The model under review builds one solid part; all positions refer to its coordinate system, in mm. Face numbers are marked on the shaded views. A direction names the side the tool comes from. Round coordinates to 2 decimals unless told otherwise and drop trailing zeros. Order: outer loops, then holes, each group sorted by start corner. A loop starts at its lowest first (then second) coordinate and runs counter-clockwise, first axis right, second up. Notation, with made-up numbers: M 50.5,70.5 L 59.5,70.5 A15 ccw 59.5,92.5 Z; hole C 56,34.5 d1. An arc over 180 degrees is marked long. Answer as a JSON object with one key per item and string values. Group by question number.
1) Consider section C-C, the plane x = 8. Write out the cut boundary in (y, z) (3 decimals), then the cut area to 3 significant figures.
2) For the marked faces 4, 5 and 6, list the 3-axis set-ups (+Z, -Z, +X, -X, +Y, -Y) from which the entire face can be reached by the end or side of a thin tool; tool diameter is ignored.
3) Consider section B-B, the plane z = 0. Write out the cut boundary in (x, y), then the cut area to 3 significant figures.
4) To check wall thickness, follow line 1 (X direction, y = 3.75, z = 0); line 2 (Z direction, x = 29, y = 6); line 3 (X direction, y = 2.5, z = 3). State the ranges of each line that lie inside material, in increasing order.
5) Consider section A-A, the plane y = 4. Write out the cut boundary in (x, z) (1 decimal), then the cut area to 3 significant figures.
6) The part is to be moulded in two halves that separate along X. For the marked faces 1, 2 and 3, say which applies: +X half, -X half, draft (parallel to the pull), parting line (faces both ways), or undercut.
7) Insertion check: pin 1 Ø3.5 at (x, y) = (16, 5) entering from +Z (3 decimals); pin 2 Ø2 at (x, z) = (18.5, 4) entering from -Y; pin 3 Ø5.5 at (x, z) = (29, 0) entering from +Y; pin 4 Ø1 at (x, y) = (14.5, 5.5) entering from -Z (3 decimals). Each pin has a flat end and moves straight along its axis. Give the tip position at first contact, or say it passes through.
```python
from build123d import *

# Parameters (mm, degrees)
SKETCH1_R           = 5
BOSS_EXTRUDE1_DEPTH = 10
FILLET1_R           = 2.54
SCALE1_SCALE        = 0.66


with BuildPart() as part:
    # Sketch1 → Boss-Extrude1 (new body)
    with BuildSketch(Plane(origin=(0, 0, 0), x_dir=(1, 0, 0), z_dir=(0, 1, 0))):
        with BuildLine():
            Line((-0.840776184, -6.25), (25.840776184, -6.25))
            ThreePointArc((25.840776184, -6.25), (28.902638362, -6.730283618), (31.670388092, -8.125))
            ThreePointArc((31.670388092, -8.125), (47.5, 0), (31.670388092, 8.125))
            ThreePointArc((31.670388092, 8.125), (28.902638362, 6.730283618), (25.840776184, 6.25))
            Line((25.840776184, 6.25), (-0.840776184, 6.25))
            ThreePointArc((-0.840776184, 6.25), (-3.902638362, 6.730283618), (-6.670388092, 8.125))
            ThreePointArc((-6.670388092, 8.125), (-22.5, 0), (-6.670388092, -8.125))
            ThreePointArc((-6.670388092, -8.125), (-3.902638362, -6.730283618), (-0.840776184, -6.25))
        make_face()
        with Locations((-12.5, 0)):
            Circle(SKETCH1_R, mode=Mode.SUBTRACT)
        with Locations((37.5, 0)):
            Circle(SKETCH1_R, mode=Mode.SUBTRACT)
    extrude(amount=BOSS_EXTRUDE1_DEPTH)

    # Fillet1
    fillet1_edges = [part.edges().sort_by_distance(p)[0] for p in [
        (-3.902638362, 10, 6.730283618),
        (-22.5, 0, 0),
        (-3.902638362, 0, -6.730283618),
        (12.5, 10, 6.25),
        (28.902638362, 10, 6.730283618),
        (47.5, 10, 0),
        (28.902638362, 10, -6.730283618),
        (12.5, 10, -6.25),
        (-3.902638362, 10, -6.730283618),
        (-22.5, 10, 0),
        (12.5, 0, -6.25),
        (28.902638362, 0, -6.730283618),
        (47.5, 0, 0),
        (28.902638362, 0, 6.730283618),
        (12.5, 0, 6.25),
        (-3.902638362, 0, 6.730283618),
    ]]
    fillet(fillet1_edges, radius=FILLET1_R)


with BuildPart() as part_1:
    # Scale1: scaled about (12.5, 5, 0)
    add(part.part.scale(SCALE1_SCALE).moved(Location((4.25, 1.7, 0))))


solid = part_1.part
```
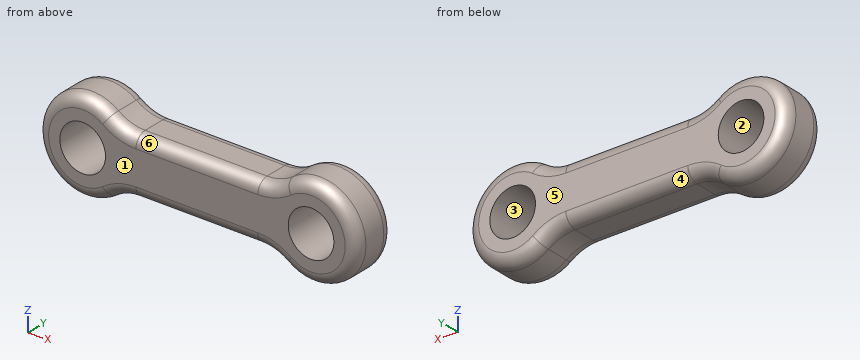
Results list:
{
 "1": {"outline": "M 1.7,-2.449 A1.676 ccw 3.376,-4.125 L 6.624,-4.125 A1.676 ccw 8.3,-2.449 L 8.3,2.449 A1.676 ccw 6.624,4.125 L 3.376,4.125 A1.676 ccw 1.7,2.449 Z", "area": "52.0 mm^2"},
 "2": {"face 4": "-Z, +Y", "face 5": "+Z, -Z, +X, -X, +Y", "face 6": "+Z, -Y"},
 "3": {"outline": "M -10.6,3.38 A1.68 ccw -8.92,1.7 L -7.3,1.7 L -7.3,8.3 L -8.92,8.3 A1.68 ccw -10.6,6.62 Z; M -0.7,1.7 L 25.7,1.7 L 25.7,8.3 L -0.7,8.3 Z; M 32.3,1.7 L 33.92,1.7 A1.68 ccw 35.6,3.38 L 35.6,6.62 A1.68 ccw 33.92,8.3 L 32.3,8.3 Z", "area": "215 mm^2"},
 "4": {"line 1": "-10.6 to -7.3, -0.7 to 25.7, 32.3 to 35.6", "line 2": "-6.6 to -3.3, 3.3 to 6.6", "line 3": "-9.6 to -5.37, -2.63 to 27.63, 30.37 to 34.6"},
 "5": {"outline": "M -0.2,-5.4 A6.6 cw 3.7,-4.1 L 21.3,-4.1 A6.6 cw 25.2,-5.4 A6.6 ccw long 25.2,5.4 A6.6 cw 21.3,4.1 L 3.7,4.1 A6.6 cw -0.2,5.4 A6.6 ccw long Z; hole C -4,0 d6.6; hole C 29,0 d6.6", "area": "379 mm^2"},
 "6": {"face 1": "draft", "face 2": "undercut", "face 3": "undercut"},
 "7": {"pin 1": "z = 4.125", "pin 2": "y = 1.79", "pin 3": "through", "pin 4": "z = -4.125"}
}
